from build123d import *

# Parameters (mm, degrees)
SKETCH1_W           = 54
SKETCH1_H           = 6.75
SKETCH1_R           = 1.1
BOSS_EXTRUDE1_DEPTH = 3
FILLET1_R           = 0.5


with BuildPart() as part:
    # Sketch1 → Boss-Extrude1 (new body)
    with BuildSketch(Plane(origin=(0, 0, 0), x_dir=(1, 0, 0), z_dir=(0, 1, 0))):
        Rectangle(SKETCH1_W, SKETCH1_H)
        with Locations(Location((-23.5, 0, 0), (0, 0, 270))):
            Circle(SKETCH1_R, mode=Mode.SUBTRACT)
        with Locations(Location((23.5, 0, 0), (0, 0, 270))):
            Circle(SKETCH1_R, mode=Mode.SUBTRACT)
    extrude(amount=BOSS_EXTRUDE1_DEPTH)

    # Fillet1
    fillet1_edges = [part.edges().sort_by_distance(p)[0] for p in [
        (-27, 3, 0),
        (0, 3, 3.375),
        (27, 3, 0),
        (0, 0, 3.375),
        (-27, 0, 0),
        (0, 0, -3.375),
        (27, 0, 0),
        (27, 1.5, 3.375),
        (-27, 1.5, 3.375),
        (-27, 1.5, -3.375),
        (27, 1.5, -3.375),
        (0, 3, -3.375),
    ]]
    fillet(fillet1_edges, radius=FILLET1_R)


solid = part.part
Could you check a few things on this model? Use its own coordinates, in mm. Give positions to 0.01 mm unless a question says otherwise; leave off trailing zeros. Order: outer loops, then holes, each group sorted by start corner. A loop starts at its lowest first (then second) coordinate and runs counter-clockwise, first axis right, second up. Notation, with made-up numbers: (52.5, 87) - (59.5, 87) arc R16 cw to (59.5, 114) - close; hole circle Ø10 at (11, -14). An arc over 180 degrees is marked (long way). One line per question, with ' | ' between items. Start each with the question number.
Item 1: Thinking about a two-plate mould opening in Z: for faces 1 (the cylindrical face through (-24.574, 1.479, -0.238)), 2 (the flat face through (0, 0, 0)), 3 (the flat face through (0, 1, 3.375)), which applies, pulls with the +Z half, pulls with the -Z half, needs draft (parallel to the pull), parting line crosses it, or undercut?
Item 2: I want a section at A-A on x = 23.5. Write out the boundary of the cut face in (y, z) (3 decimals), then the cut area to 3 significant figures.
Item 3: I want a section at B-B on y = 1.1. Write out the boundary of the cut face in (x, z) (3 decimals), then the cut area to 3 significant figures.
Item 4: I need wall thicknesses on probe 1 along X at (y, z) = (0.85, 0); probe 2 along X at (y, z) = (0.85, -1); probe 3 along Z at (x, y) = (-22.5, 1.85) (3 decimals). Which ranges of each line are inside material? Lowest first, please. Write a range as [from, to].
Verdict:
1) face 1: undercut | face 2: needs draft | face 3: pulls with the +Z half
2) outline: (0, -2.875) arc R0.5 ccw to (0.5, -3.375) - (2.5, -3.375) arc R0.5 ccw to (3, -2.875) - (3, -1.1) - (0, -1.1) - close; (0, 1.1) - (3, 1.1) - (3, 2.875) arc R0.5 ccw to (2.5, 3.375) - (0.5, 3.375) arc R0.5 ccw to (0, 2.875) - close | area: 13.4 mm^2
3) outline: (-27, -2.875) arc R0.5 ccw to (-26.5, -3.375) - (26.5, -3.375) arc R0.5 ccw to (27, -2.875) - (27, 2.875) arc R0.5 ccw to (26.5, 3.375) - (-26.5, 3.375) arc R0.5 ccw to (-27, 2.875) - close; hole circle Ø2.2 at (-23.5, 0); hole circle Ø2.2 at (23.5, 0) | area: 357 mm^2
4) probe 1: [-27, -24.6], [-22.4, 22.4], [24.6, 27] | probe 2: [-27, -23.96], [-23.04, 23.04], [23.96, 27] | probe 3: [-3.375, -0.458], [0.458, 3.375]
